Build history of the part. All positions in model axes, mm. Give positions to 0.01 mm unless a question says otherwise; leave off trailing zeros. Order: outer loops, then holes, each group sorted by start corner. A loop starts at its lowest first (then second) coordinate and runs counter-clockwise, first axis right, second up. Notation, with made-up numbers: (-13.5, 71) - (14.5, 71) arc R27 cw to (14.5, 101) - close; hole circle Ø5 at (58, -21.75). An arc over 180 degrees is marked (long way). Use a Markdown table: item, result. Add a question column.
(1) Slice it at A-A (x = 69.5). Write the cut outline in (y, z).
(2) Wall check: line 1 (Y direction, x = 72, z = 1.25); line 2 (Z direction, x = 47.5, y = 100.5); line 3 (X direction, y = 338, z = 0.5). Give the ranges that are in metal, low to high.
(3) Slice it at B-B (y = 159). Write the cut outline in (x, z).
(4) Slice it at C-C (z = -5). Write the cut outline in (x, y), then the cut area to 3 significant figures.
(5) Flat gauge pins, fed straight in: pin 1 (0.9 mm diameter, centred on x = 90, z = 1, fed in from +Y); pin 2 (0.9 mm diameter, centred on x = -2, z = 1.5, fed in from -Y); pin 3 (6 mm diameter, centred on y = 282, z = -6.5, fed in from -X). Where does each tip first touch, or does it go through?
(6) Slice it at D-D (y = 261.5). Write the cut outline in (x, z), then the cut area to 3 significant figures.
Autodesk Inventor part; units mm, degrees
ref_plane "YZ Plane" through (0, 0, 0) normal (1, 0, 0) x (0, 1, 0)
ref_plane "XZ Plane" through (0, 0, 0) normal (0, 1, 0) x (-1, 0, 0)
ref_plane "XY Plane" through (0, 0, 0) normal (0, 0, 1) x (1, 0, 0)
sketch "Sketch1" plane through (0, 0, 0) normal (0, 0, 1) x (1, 0, 0)
  line L0 (0, 0) -> (88, 0)
  line L1 (88, 0) -> (88, 10)
  line L2 (88, 10) -> (91, 10)
  line L3 (91, 10) -> (91, 30)
  line L4 (91, 30) -> (88, 30)
  line L5 (88, 30) -> (88, 50)
  line L6 (88, 50) -> (91, 50)
  line L7 (91, 50) -> (91, 70)
  line L8 (91, 70) -> (88, 70)
  line L9 (88, 70) -> (88, 90)
  line L10 (88, 90) -> (91, 90)
  line L11 (91, 90) -> (91, 110)
  line L12 (91, 110) -> (88, 110)
  line L13 (88, 110) -> (88, 130)
  line L14 (88, 130) -> (91, 130)
  line L15 (91, 130) -> (91, 150)
  line L16 (91, 150) -> (88, 150)
  line L17 (88, 150) -> (88, 170)
  line L18 (88, 170) -> (91, 170)
  line L19 (91, 170) -> (91, 190)
  line L20 (91, 190) -> (88, 190)
  line L21 (88, 190) -> (88, 210)
  line L22 (88, 210) -> (91, 210)
  line L23 (91, 210) -> (91, 230)
  line L24 (91, 230) -> (88, 230)
  line L25 (88, 230) -> (88, 250)
  line L26 (88, 250) -> (91, 250)
  line L27 (91, 250) -> (91, 270)
  line L28 (91, 270) -> (88, 270)
  line L29 (88, 270) -> (88, 290)
  line L30 (88, 290) -> (91, 290)
  line L31 (91, 290) -> (91, 310)
  line L32 (91, 310) -> (88, 310)
  line L33 (88, 310) -> (88, 330)
  line L34 (88, 330) -> (91, 330)
  line L35 (91, 330) -> (91, 350)
  line L36 (91, 350) -> (88, 350)
  line L37 (88, 350) -> (88, 370)
  line L38 (88, 370) -> (91, 370)
  line L39 (91, 370) -> (91, 390)
  line L40 (91, 390) -> (88, 390)
  line L41 (88, 390) -> (88, 410)
  line L42 (88, 410) -> (91, 410)
  line L43 (91, 410) -> (91, 430)
  line L44 (91, 430) -> (88, 430)
  line L45 (44, 0) -> (44, 110) construction
  line L46 (-3, 10) -> (-3, 30)
  line L47 (-3, 30) -> (0, 30)
  line L48 (0, 10) -> (-3, 10)
  line L49 (0, 50) -> (-3, 50)
  line L50 (-3, 50) -> (-3, 70)
  line L51 (0, 70) -> (0, 90)
  line L52 (0, 90) -> (-3, 90)
  line L53 (-3, 90) -> (-3, 110)
  line L54 (-3, 70) -> (0, 70)
  line L55 (-3, 110) -> (0, 110)
  line L56 (0, 110) -> (0, 130)
  line L57 (0, 130) -> (-3, 130)
  line L58 (-3, 130) -> (-3, 150)
  line L59 (-3, 170) -> (-3, 190)
  line L60 (0, 150) -> (0, 170)
  line L61 (0, 170) -> (-3, 170)
  line L62 (-3, 150) -> (0, 150)
  line L63 (0, 190) -> (0, 210)
  line L64 (-3, 190) -> (0, 190)
  line L65 (0, 210) -> (-3, 210)
  line L66 (-3, 210) -> (-3, 230)
  line L67 (-3, 230) -> (0, 230)
  line L68 (0, 230) -> (0, 250)
  line L69 (0, 250) -> (-3, 250)
  line L70 (-3, 250) -> (-3, 270)
  line L71 (-3, 270) -> (0, 270)
  line L72 (0, 270) -> (0, 290)
  line L73 (0, 290) -> (-3, 290)
  line L74 (-3, 290) -> (-3, 310)
  line L75 (-3, 310) -> (0, 310)
  line L76 (0, 310) -> (0, 330)
  line L77 (0, 350) -> (0, 370)
  line L78 (-3, 350) -> (0, 350)
  line L79 (-3, 330) -> (-3, 350)
  line L80 (0, 330) -> (-3, 330)
  line L81 (0, 370) -> (-3, 370)
  line L82 (-3, 370) -> (-3, 390)
  line L83 (-3, 390) -> (0, 390)
  line L84 (0, 390) -> (0, 410)
  line L85 (0, 410) -> (-3, 410)
  line L86 (-3, 410) -> (-3, 430)
  line L87 (-3, 430) -> (0, 430)
  line L88 (0, 430) -> (0, 450)
  line L89 (0, 450) -> (88, 450)
  line L90 (88, 430) -> (88, 450)
  line L91 (0, 50) -> (0, 30)
  line L92 (0, 10) -> (0, 0)
  point P0 (0, 0)
  dimension "d1" = 10
  dimension "d2" = 3
  dimension "d3" = 20
  dimension "d4" = 3
  dimension "d5" = 20
  dimension "d6" = 20
  dimension "d7" = 20
  dimension "d8" = 20
  dimension "d9" = 20
  dimension "d10" = 3
  dimension "d11" = 20
  dimension "d12" = 20
  dimension "d13" = 20
  dimension "d14" = 3
  dimension "d15" = 20
  dimension "d16" = 3
  dimension "d17" = 20
  dimension "d18" = 20
  dimension "d19" = 20
  dimension "d20" = 3
  dimension "d21" = 20
  dimension "d22" = 20
  dimension "d23" = 20
  dimension "d24" = 20
  dimension "d25" = 20
  dimension "d26" = 20
  dimension "d27" = 20
  dimension "d28" = 20
  dimension "d30" = 0
  dimension "d31" = 0
  dimension "d34" = 110
  dimension "d35" = 0
  dimension "d36" = 0
  dimension "d37" = 0
  dimension "d38" = 0
  dimension "d39" = 3
  dimension "d43" = 88
  dimension "d65" = 20
extrude "Extrusion1" add sketch "Sketch1" along normal blind 3
sketch "Sketch4" plane through (0, 0, 0) normal (0, 0, -1) x (-1, 0, 0)
  line L0 (-98.5, 430) -> (-44, 430)
  line L1 (-91, 430) -> (3, 430)
  line L2 (-44.5, 330) -> (-75, 330)
  line L3 (-75, 350) -> (-75, 0)
  line L4 (-75, 330) -> (-75, 370)
  line L5 (-75, 370) -> (-43, 370)
  line L6 (-43, 370) -> (-13, 370)
  line L7 (-13, 370) -> (-13, 330)
  line L8 (-13, 330) -> (-44.5, 330)
  line L9 (0, 370) -> (0, 350)
  point P0 (0, 0)
  dimension "d55" = 30
  dimension "d58" = 60
  dimension "d59" = 40
  dimension "d61" = 30.5
  dimension "d62" = 0
  dimension "d63" = 80
  dimension "d64" = 23.5
  dimension "d66" = 13
extrude "Extrusion4" cut sketch "Sketch4" against normal blind 19
sketch "Sketch5" plane through (0, 0, 3) normal (0, 0, 1) x (1, 0, 0)
  point P0 (0, 0)
sketch "Sketch6" plane through (0, 0, 0) normal (0, 0, -1) x (-1, 0, 0)
  line L0 (0, 0) -> (-88, 0)
  line L1 (-44, 0) -> (-44, 330)
  line L2 (-75, 330) -> (-13, 330)
  line L3 (-44, 0) -> (-42.5, 0)
  line L4 (-42.5, 0) -> (-42.5, 330)
  line L5 (-44, 330) -> (-45.5, 330)
  line L6 (-45.5, 330) -> (-45.5, 0)
  line L7 (-44, 0) -> (-45.5, 0)
  dimension "d67" = 1.5
  dimension "d68" = 1.5
extrude "Extrusion5" add sketch "Sketch6" along normal blind 8
ref_plane "Work Plane1" through (44, 430, 0) normal (1, 0, 0) x (0, 0, -1)
properties part number "Part4 box" material "Wood (Birch)"
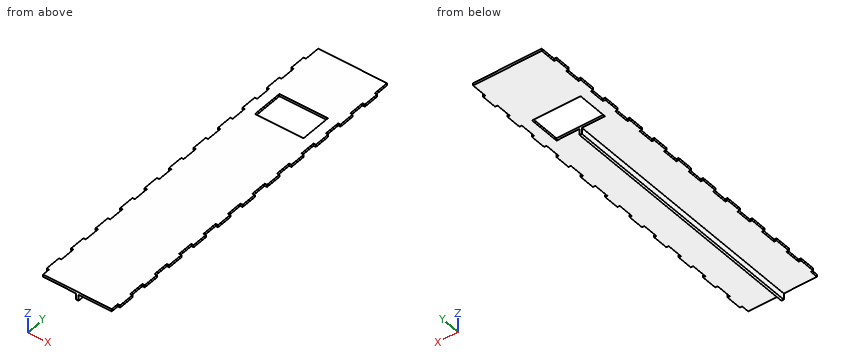
Solution:
| question | item | result |
|---|---|---|
| 1 | outline | (0, 0) - (330, 0) - (330, 3) - (0, 3) - close; (370, 0) - (450, 0) - (450, 3) - (370, 3) - close |
| 2 | line 1 | 0 to 330, 370 to 450 |
| 2 | line 2 | 0 to 3 |
| 2 | line 3 | -3 to 13, 75 to 91 |
| 3 | outline | (0, 0) - (42.5, 0) - (42.5, -8) - (45.5, -8) - (45.5, 0) - (88, 0) - (88, 3) - (0, 3) - close |
| 4 | outline | (42.5, 0) - (45.5, 0) - (45.5, 330) - (42.5, 330) - close |
| 4 | area | 990 mm2 |
| 5 | pin 1 | y = 430 |
| 5 | pin 2 | y = 10 |
| 5 | pin 3 | x = 42.5 |
| 6 | outline | (-3, 0) - (42.5, 0) - (42.5, -8) - (45.5, -8) - (45.5, 0) - (91, 0) - (91, 3) - (-3, 3) - close |
| 6 | area | 306 mm2 |
